Geometry: final body of the model. Coordinates: model frame, mm. Face numbers are marked on the shaded views. A direction names the side the tool comes from. Coordinates: 2 decimals unless noted, no trailing zeros. Order: outer loops, then holes, each group sorted by start corner. A loop starts at its lowest first (then second) coordinate and runs counter-clockwise, first axis right, second up. Notation, with made-up numbers: M 81,-13 L 101,-13 A12 ccw 101,-4 Z; hole C -2.75,-8 d1. An arc over 180 degrees is marked long. Use CSV: the item, a comma, the result in double quotes. Start each with the question number.
Q1. Ray query, probe 1 along X at (y, z) = (-16.5, 1.1); probe 2 along Y at (x, z) = (0, 2.25). Return the intervals inside material, ascending.
Q2. Section query A-A, the plane x = 0. Output: boundary loops of the cut face in (y, z) (1 decimal).
Q3. Mould query, pull axis X, two halves, no side actions, for the marked faces 4, 5 and 6. Classes: +X half, -X half, draft (parallel to the pull), parting line (faces both ways), or undercut.
Q4. Section query C-C, the plane y = -13.5. Output: boundary loops of the cut face in (x, z) (3 decimals), and give its area (3 significant figures).
Q5. Access query for the marked faces 1, 2 and 3. Directions: +Z, -Z, +X, -X, +Y, -Y. A direction counts if a zero-diameter tool reaches every point of the face in a straight line with its end or side. Return the directions, or none.
Q6. First-contact query: P1, Ø1.6, axis at y = -12, z = 1, coming from the +X side; P2, Ø1.6, axis at y = 16.5, z = 1.5, coming from the +X side; P3, Ø1, axis at x = 17, z = 2, coming from the -Y side. Flat tips, straight axial feed; report the tip coordinate or a pass-through.
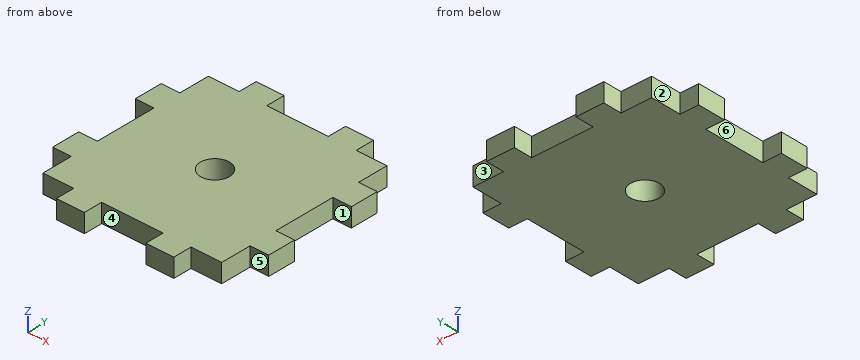
from build123d import *

# Parameters (mm, degrees)
F0_W     = 2.38125
F0_H     = 3.175
F0_W_2   = 3.175
F0_H_2   = 2.38125
F0_W_3   = 7.62
F0_H_3   = 7.62
F1_DEPTH = 3.175
F2_R     = 2.4765
F3_DEPTH = 25.4


with BuildPart() as f1:
    # F0 (on Top) → F1 (new body)
    with BuildSketch(Plane.XY):
        Polygon((-7.62, 15.24), (-5.23875, 15.24), (-5.23875, 18.415), (-10.00125, 18.415), (-10.00125, 15.24), align=None)
        with Locations((-8.810625, 13.6525)):
            Rectangle(F0_W, F0_H)
        with Locations((-6.429375, 13.6525)):
            Rectangle(F0_W, F0_H)
        Polygon((0, 7.62), (0, 15.24), (-5.23875, 15.24), (-5.23875, 12.065), (-7.62, 12.065), (-7.62, 7.62), align=None)
        Polygon((-12.065, 7.62), (-7.62, 7.62), (-7.62, 12.065), (-10.00125, 12.065), (-10.00125, 15.24), (-15.24, 15.24), (-15.24, 10.00125), (-12.065, 10.00125), align=None)
        with Locations((-13.6525, 8.810625)):
            Rectangle(F0_W_2, F0_H_2)
        with Locations((-13.6525, 6.429375)):
            Rectangle(F0_W_2, F0_H_2)
        Polygon((-15.24, 5.23875), (-15.24, 7.62), (-15.24, 10.00125), (-18.415, 10.00125), (-18.415, 5.23875), align=None)
        Polygon((-7.62, 0), (-7.62, 7.62), (-12.065, 7.62), (-12.065, 5.23875), (-15.24, 5.23875), (-15.24, 0), align=None)
        with Locations((-3.81, 3.81)):
            Rectangle(F0_W_3, F0_H_3)
        with Locations((3.81, 3.81)):
            Rectangle(F0_W_3, F0_H_3)
        Polygon((5.23875, 12.065), (5.23875, 15.24), (0, 15.24), (0, 7.62), (7.62, 7.62), (7.62, 12.065), align=None)
        with Locations((6.429375, 13.6525)):
            Rectangle(F0_W, F0_H)
        with Locations((8.810625, 13.6525)):
            Rectangle(F0_W, F0_H)
        Polygon((7.62, 15.24), (10.00125, 15.24), (10.00125, 18.415), (5.23875, 18.415), (5.23875, 15.24), align=None)
        Polygon((15.24, 0), (15.24, 5.23875), (12.065, 5.23875), (12.065, 7.62), (7.62, 7.62), (7.62, 0), align=None)
        Polygon((15.24, 10.00125), (15.24, 15.24), (10.00125, 15.24), (10.00125, 12.065), (7.62, 12.065), (7.62, 7.62), (12.065, 7.62), (12.065, 10.00125), align=None)
        with Locations((13.6525, 8.810625)):
            Rectangle(F0_W_2, F0_H_2)
        with Locations((13.6525, 6.429375)):
            Rectangle(F0_W_2, F0_H_2)
        Polygon((18.415, 10.00125), (15.24, 10.00125), (15.24, 7.62), (15.24, 5.23875), (18.415, 5.23875), align=None)
        Polygon((15.24, -5.23875), (15.24, 0), (7.62, 0), (7.62, -7.62), (12.065, -7.62), (12.065, -5.23875), align=None)
        with Locations((13.6525, -6.429375)):
            Rectangle(F0_W_2, F0_H_2)
        Polygon((12.065, -7.62), (7.62, -7.62), (7.62, -12.065), (10.00125, -12.065), (10.00125, -15.24), (15.24, -15.24), (15.24, -10.00125), (12.065, -10.00125), align=None)
        Polygon((18.415, -5.23875), (15.24, -5.23875), (15.24, -7.62), (15.24, -10.00125), (18.415, -10.00125), align=None)
        with Locations((13.6525, -8.810625)):
            Rectangle(F0_W_2, F0_H_2)
        with Locations((6.429375, -13.6525)):
            Rectangle(F0_W, F0_H)
        with Locations((8.810625, -13.6525)):
            Rectangle(F0_W, F0_H)
        Polygon((10.00125, -15.24), (7.62, -15.24), (5.23875, -15.24), (5.23875, -18.415), (10.00125, -18.415), align=None)
        Polygon((7.62, -12.065), (7.62, -7.62), (0, -7.62), (0, -15.24), (5.23875, -15.24), (5.23875, -12.065), align=None)
        with Locations((3.81, -3.81)):
            Rectangle(F0_W_3, F0_H_3)
        with Locations((-3.81, -3.81)):
            Rectangle(F0_W_3, F0_H_3)
        Polygon((-7.62, -7.62), (-7.62, 0), (-15.24, 0), (-15.24, -5.23875), (-12.065, -5.23875), (-12.065, -7.62), align=None)
        with Locations((-13.6525, -6.429375)):
            Rectangle(F0_W_2, F0_H_2)
        with Locations((-13.6525, -8.810625)):
            Rectangle(F0_W_2, F0_H_2)
        Polygon((-15.24, -7.62), (-15.24, -5.23875), (-18.415, -5.23875), (-18.415, -10.00125), (-15.24, -10.00125), align=None)
        Polygon((-7.62, -12.065), (-7.62, -7.62), (-12.065, -7.62), (-12.065, -10.00125), (-15.24, -10.00125), (-15.24, -15.24), (-10.00125, -15.24), (-10.00125, -12.065), align=None)
        Polygon((0, -15.24), (0, -7.62), (-7.62, -7.62), (-7.62, -12.065), (-5.23875, -12.065), (-5.23875, -15.24), align=None)
        with Locations((-6.429375, -13.6525)):
            Rectangle(F0_W, F0_H)
        with Locations((-8.810625, -13.6525)):
            Rectangle(F0_W, F0_H)
        Polygon((-5.23875, -18.415), (-5.23875, -15.24), (-7.62, -15.24), (-10.00125, -15.24), (-10.00125, -18.415), align=None)
    extrude(amount=F1_DEPTH)

    # F2 (on face) → F3 (cut)
    with BuildSketch(Plane.XY.offset(3.175)):
        Circle(F2_R)
    extrude(amount=-F3_DEPTH, mode=Mode.SUBTRACT)


solid = f1.part
Responses:
1,probe 1,"x = -10 to -5.24, 5.24 to 10"
1,probe 2,"y = -15.24 to -2.48, 2.48 to 15.24"
2,outline,"M -15.2,0 L -2.5,0 L -2.5,3.2 L -15.2,3.2 Z; M 2.5,0 L 15.2,0 L 15.2,3.2 L 2.5,3.2 Z"
3,face 4,"undercut"
3,face 5,"draft"
3,face 6,"-X half"
4,outline,"M -15.24,0 L 15.24,0 L 15.24,3.175 L -15.24,3.175 Z"
4,area,"96.8 mm²"
5,face 1,"+Z, -Z, +X"
5,face 2,"+Z, -Z, -X, +Y"
5,face 3,"+Z, -Z, +X, +Y"
6,P1,"stops at x = 15.24"
6,P2,"stops at x = 10"
6,P3,"stops at y = -10"
